```python
from build123d import *

# Parameters (mm, degrees)
ESBO_O1_W                  = 74
ESBO_O1_H                  = 110
RESSALTO_EXTRUS_O1_DEPTH   = 4
FILETE1_R                  = 2
FILETE2_R                  = 2
FILETE3_R                  = 2
FILETE4_R                  = 2
CORTE_EXTRUS_O1_DEPTH      = 15
CORTE_EXTRUS_O1_DEPTH_BACK = 10
ESBO_O2_R                  = 13
CORTE_EXTRUS_O3_DEPTH      = 15
CORTE_EXTRUS_O3_DEPTH_BACK = 15
ESBO_O3_R                  = 2
ESBO_O4_R                  = 16.343681483
ESBO_O4_R_2                = 13
RESSALTO_EXTRUS_O2_DEPTH   = 10


with BuildPart() as part:
    # Esboço1 → Ressalto-extrusão1 (new body)
    with BuildSketch(Plane(origin=(0, 0, 0), x_dir=(1, 0, 0), z_dir=(0, 1, 0))):
        with Locations((27.707512014, -44.028932547)):
            Rectangle(ESBO_O1_W, ESBO_O1_H)
    extrude(amount=RESSALTO_EXTRUS_O1_DEPTH)

    # Filete1
    filete1_edges = [part.edges().sort_by_distance(p)[0] for p in [
        (27.707512014, 4, 99.028932547),
    ]]
    fillet(filete1_edges, radius=FILETE1_R)

    # Filete2
    filete2_edges = [part.edges().sort_by_distance(p)[0] for p in [
        (64.707512014, 4, 43.028932547),
        (64.707512014, 1, 99.028932547),
        (64.707512014, 3.414213562, 98.443146109),
    ]]
    fillet(filete2_edges, radius=FILETE2_R)

    # Filete3
    filete3_edges = [part.edges().sort_by_distance(p)[0] for p in [
        (64.707512014, 1, -10.971067453),
        (26.707512014, 4, -10.971067453),
        (64.121725576, 3.414213562, -10.971067453),
    ]]
    fillet(filete3_edges, radius=FILETE3_R)

    # Filete4
    filete4_edges = [part.edges().sort_by_distance(p)[0] for p in [
        (-9.292487986, 1, 99.028932547),
        (-9.292487986, 3.414213562, 98.443146109),
        (-9.292487986, 1, -10.971067453),
        (-9.292487986, 4, 44.028932547),
        (-9.292487986, 3.414213562, -10.385281015),
    ]]
    fillet(filete4_edges, radius=FILETE4_R)

    # Esboço2 → Corte-extrusão1 (cut, two sides: drawn at the far end of the back side and taken through both)
    with BuildSketch(Plane(origin=(0, 0, 0), x_dir=(1, 0, 0), z_dir=(0, 1, 0)).offset(-CORTE_EXTRUS_O1_DEPTH_BACK)):
        with Locations(Location((27.707512014, -44.028932547, 0), (0, 0, 270))):
            Circle(ESBO_O2_R)
    extrude(amount=CORTE_EXTRUS_O1_DEPTH + CORTE_EXTRUS_O1_DEPTH_BACK, mode=Mode.SUBTRACT)

    # Esboço3 → Corte-extrusão3 (cut, two sides: drawn at the far end of the back side and taken through both)
    with BuildSketch(Plane(origin=(0, 0, 0), x_dir=(1, 0, 0), z_dir=(0, 1, 0)).offset(-CORTE_EXTRUS_O3_DEPTH_BACK)):
        with Locations(Location((27.707512014, -84.328932547, 0), (0, 0, 270))):
            Circle(ESBO_O3_R)
        with Locations(Location((27.707512014, -3.728932547, 0), (0, 0, 270))):
            Circle(ESBO_O3_R)
    extrude(amount=CORTE_EXTRUS_O3_DEPTH + CORTE_EXTRUS_O3_DEPTH_BACK, mode=Mode.SUBTRACT)

    # Esboço4 → Ressalto-extrusão2 (add)
    with BuildSketch(Plane(origin=(0, 0, 0), x_dir=(1, 0, 0), z_dir=(0, 1, 0))):
        with Locations(Location((27.707512014, -44.028932547, 0), (0, 0, 270))):
            Circle(ESBO_O4_R)
        with Locations(Location((27.707512014, -44.028932547, 0), (0, 0, 270))):
            Circle(ESBO_O4_R_2, mode=Mode.SUBTRACT)
    extrude(amount=RESSALTO_EXTRUS_O2_DEPTH)


solid = part.part
```
The listing builds one solid part. Answer for the finished solid, in the listing's coordinates (mm). A direction names the side the tool comes from. Coordinates: 2 decimals unless noted, no trailing zeros. Write each loop counter-clockwise with the first axis right and the second up, starting at its lowest first coordinate (ties: lowest second). Pieces come first, ordered by that corner, then holes. Notation, with made-up numbers: M -28,21.5 L 14,21.5 A13 cw 14,28.5 Z; hole C 29,88 d7. An arc over 180 degrees is marked long. Use a Markdown table: item, result. Add a question column.
1. Section A-A (z = 23) is taken. Give the vertices of the cut face in (x, y).
2. Given P1, Ø3.5, axis at x = 27.71, z = 84.33, coming from the +Y side; P2, Ø8, axis at x = 27, z = 11, coming from the +Y side, each flat-ended and moving along its own axis, determine where each tip first touches the part or whether it passes through.
3. Section D-D (y = 5.5) is taken. Give the vertices of the cut face in (x, z), plus the area to 3 significant figures.
4. Section C-C (x = -1) is taken. Give the vertices of the cut face in (y, z), plus the area to 3 significant figures.
5. Which of the six approach directions +Z, -Z, +X, -X, +Y, -Y give full straight-line access (tool end or side, diameter ignored) to faces 1 (the flat face through (64.708, 1, 45)), 2 (the cylindrical face through (13.208, 6.958, 51.571))?
6. Section B-B (x = 33) is taken. Give the vertices of the cut face in (y, z), plus the area to 3 significant figures.
7. Straight lines are drawn through the part: line 1 along Y through (x, z) = (7.5, 58); line 2 along X through (y, z) = (5.75, 54); line 3 along Z through (x, y) = (33, 8). For each, find the intervals that lie inside material, in ascending order. Write a range as [from, to].
8. For a pull along Z with two mould halves and no side action, classify faces 3 (the cylindrical face through (-8.72, 3.4, 43.29)), 4 (the cylindrical face through (64.106, 1.014, 98.459)), 5 (the cylindrical face through (27.8, 1.97, 82.33)) as +Z half, -Z half, draft (parallel to the pull), parting line (faces both ways), or undercut.
Data:
| question | item | result |
|---|---|---|
| 1 | outline | M -9.29,0 L 64.71,0 L 64.71,2 A2 ccw 62.71,4 L -7.29,4 A2 ccw -9.29,2 Z |
| 2 | P1 | passes through |
| 2 | P2 | stops at y = 4 |
| 3 | outline | C 27.71,44.03 d32.69; hole C 27.71,44.03 d26 |
| 3 | area | 308 mm2 |
| 4 | outline | M 0,-10.97 L 2,-10.97 A2 ccw 4,-8.97 L 4,97.03 A2 ccw 2,99.03 L 0,99.03 Z |
| 4 | area | 438 mm2 |
| 5 | face 1 | +Z, -Z, +X, +Y, -Y |
| 5 | face 2 | +Y |
| 6 | outline | M 0,-10.97 L 2,-10.97 A2 ccw 4,-8.97 L 4,28.57 L 10,28.57 L 10,32.16 L 0,32.16 Z; M 0,55.9 L 10,55.9 L 10,59.49 L 4,59.49 L 4,97.03 A2 ccw 2,99.03 L 0,99.03 Z |
| 6 | area | 386 mm2 |
| 7 | line 1 | y = [0, 4] |
| 7 | line 2 | x = [14.76, 19.37], [36.05, 40.66] |
| 7 | line 3 | z = [28.57, 32.16], [55.9, 59.49] |
| 8 | face 3 | draft |
| 8 | face 4 | +Z half |
| 8 | face 5 | undercut |
